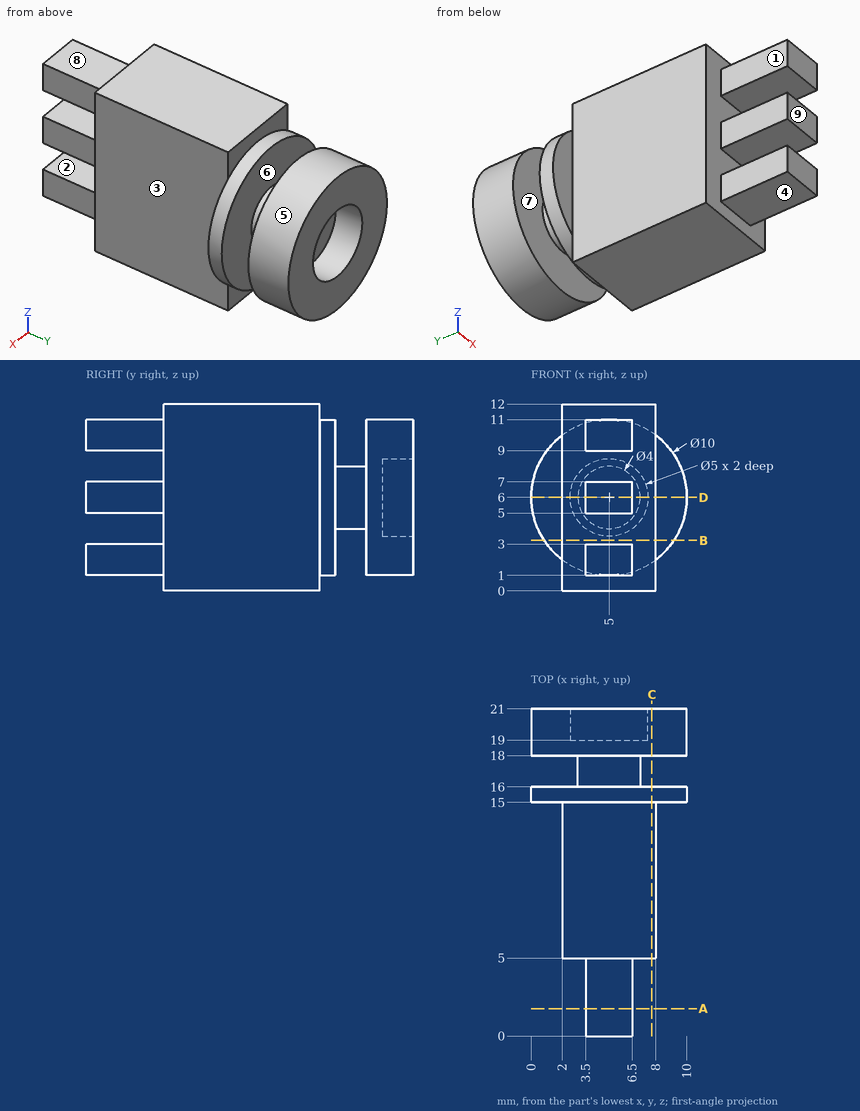
Job drawing, mm, ordinate dimensions from the low corner. One solid piece. A direction names the side the tool comes from. Coordinates: 2 decimals unless noted, no trailing zeros. Write each loop counter-clockwise with the first axis right and the second up, starting at its lowest first coordinate (ties: lowest second). Pieces come first, ordered by that corner, then holes. Notation, with made-up numbers: (-35.75, -3) - (12.25, -3) arc R27 ccw to (12.25, 30) - close; hole circle Ø4 at (-18, 19). An arc over 180 degrees is marked (long way). Use a Markdown table: item, result. Add a question column.
Item 1: Band-saw the part on B-B, the plane z = 3.25. Give the cut face in (x, y).
Item 2: Flat gauge pins, fed straight in: pin 1 (0.6 mm diameter, centred on x = 4, z = 0.5, fed in from +Y); pin 2 (3.5 mm diameter, centred on x = 5.5, y = 2, fed in from -Z); pin 3 (0.6 mm diameter, centred on y = 1.5, z = 10, fed in from -X). Where does each tip first touch, or does it go through?
Item 3: Mould opens along Y. For the marked faces 6, 7, 8 and 9 say: pulls with the +Y half, pulls with the -Y half, needs draft (parallel to the pull), parting line crosses it, or undercut.
Item 4: Band-saw the part on D-D, the plane z = 6. Give the cut face in (x, y).
Item 5: 3-axis set-ups, long thin cutter, end or side, ignore diameter. For the marked faces 1, 2, 3, 4 and 5: which of +Z, -Z, +X, -X, +Y, -Y reach the whole face in a straight line?
Item 6: Band-saw the part on A-A, the plane y = 1.75. Give the cut face in (x, z).
Item 7: Band-saw the part on C-C, the plane x = 7.75. Give the cut face in (y, z), and give its area (3 significant figures).
Item 8: Drill centre lines: L1, parallel to Y at x = 4.75, z = 10; L2, parallel to Z at x = 5, y = 19.8; L3, parallel to Y at x = 2.5, z = 2.5. Where is each one in solid material? Low to high. Write a range as from..to.
Numbers:
| question | item | result |
|---|---|---|
| 1 | outline | (0.82, 15) - (2, 15) - (2, 5) - (8, 5) - (8, 15) - (9.18, 15) - (9.18, 16) - (0.82, 16) - close; (0.82, 18) - (9.18, 18) - (9.18, 21) - (0.82, 21) - close |
| 2 | pin 1 | y = 15 |
| 2 | pin 2 | z = 1 |
| 2 | pin 3 | x = 3.5 |
| 3 | face 6 | undercut |
| 3 | face 7 | undercut |
| 3 | face 8 | needs draft |
| 3 | face 9 | pulls with the -Y half |
| 4 | outline | (0, 15) - (2, 15) - (2, 5) - (3.5, 5) - (3.5, 0) - (6.5, 0) - (6.5, 5) - (8, 5) - (8, 15) - (10, 15) - (10, 16) - (7, 16) - (7, 18) - (10, 18) - (10, 21) - (7.5, 21) - (7.5, 19) - (2.5, 19) - (2.5, 21) - (0, 21) - (0, 18) - (3, 18) - (3, 16) - (0, 16) - close |
| 5 | face 1 | +Z, -Z, -X, -Y |
| 5 | face 2 | +X, -X, -Y |
| 5 | face 3 | +Z, -Z, +X, -Y |
| 5 | face 4 | -Z, +X, -X, -Y |
| 5 | face 5 | +Y |
| 6 | outline | (3.5, 1) - (6.5, 1) - (6.5, 3) - (3.5, 3) - close; (3.5, 5) - (6.5, 5) - (6.5, 7) - (3.5, 7) - close; (3.5, 9) - (6.5, 9) - (6.5, 11) - (3.5, 11) - close |
| 7 | outline | (5, 0) - (15, 0) - (15, 1.82) - (16, 1.82) - (16, 10.18) - (15, 10.18) - (15, 12) - (5, 12) - close; (18, 1.82) - (21, 1.82) - (21, 10.18) - (18, 10.18) - close |
| 7 | area | 153 mm2 |
| 8 | L1 | 0..16, 18..21 |
| 8 | L2 | 1..3.5, 8.5..11 |
| 8 | L3 | 5..16, 18..21 |
